Autodesk Inventor part; units mm, degrees
ref_plane "YZ Plane" through (0, 0, 0) normal (1, 0, 0) x (0, 1, 0)
ref_plane "XZ Plane" through (0, 0, 0) normal (0, 1, 0) x (-1, 0, 0)
ref_plane "XY Plane" through (0, 0, 0) normal (0, 0, 1) x (1, 0, 0)
sketch "Sketch2" plane through (0, 0, 0) normal (0, 1, 0) x (-1, 0, 0)
  circle A0 centre (0, 0) radius 30.16 construction
  line L0 (0, 0) -> (38.16, 0) construction
  line L1 (38.16, 38.16) -> (38.16, -38.16)
  line L2 (38.16, 38.16) -> (-30.16, 38.16)
  line L3 (38.16, -38.16) -> (-30.16, -38.16)
  circle A1 centre (27.211, 31.78) radius 2.55
  circle A2 centre (27.211, -31.78) radius 2.55
  circle A3 centre (0, 0) radius 2.55
  line L4 (-30.16, 38.16) -> (-30.16, -38.16)
  dimension "d12" = 60.32
  dimension "d13" = 38.16
  dimension "d14" = 76.32
  dimension "d15" = 5.1
  dimension "d17" = 6.38
  dimension "d18" = 10.949
  dimension "d19" = 5.1
extrude "Extrusion2" add sketch "Sketch2" along normal blind 3
fillet "Fillet2" radius 3 2 edges at (-38.16, 1.5, 38.16) (-38.16, 1.5, -38.16)
properties part number "Tapa" material "PMMA Plastic"
Source: CAD feature listing. Evaluate the final solid. Frame: model axes, mm. Round coordinates to 2 decimals unless told otherwise and drop trailing zeros. Order: outer loops, then holes, each group sorted by start corner. A loop starts at its lowest first (then second) coordinate and runs counter-clockwise, first axis right, second up. Notation, with made-up numbers: (78.25, -31) - (118.25, -31) arc R26 cw to (118.25, -8) - close; hole circle Ø10 at (24.25, 46). An arc over 180 degrees is marked (long way). Use a Markdown table: item, result. Add a question column.
1. First-contact query: pin 1 (4.5 mm diameter, centred on x = -27.211, z = 31.78, fed in from +Y). Flat tip, straight axial feed; report the tip coordinate or a pass-through.
2. Mould query, pull axis Z, two halves, no side actions, for faces 1 (the cylindrical face through (-37.3, 1.52, 37.26)), 2 (the cylindrical face through (-37.26, 1.52, -37.3)), 3 (the flat face through (30.16, 1, 1)), 4 (the cylindrical face through (-25.33, 1.48, 30.06)). Classes: +Z half, -Z half, draft (parallel to the pull), parting line (faces both ways), or undercut.
3. Line query: probe 1 along Z at (x, y) = (0, 0.95); probe 2 along Z at (x, y) = (-25, 1.3); probe 3 along Z at (x, y) = (-1, 2.45). Output: solid intervals per line, ascending.
4. Section query A-A (z = 31.78). Return the cut outline in (x, y), then the cut area to 3 significant figures.
Derived:
| question | item | result |
|---|---|---|
| 1 | pin 1 | through |
| 2 | face 1 | +Z half |
| 2 | face 2 | -Z half |
| 2 | face 3 | draft |
| 2 | face 4 | undercut |
| 3 | probe 1 | -38.16 to -2.55, 2.55 to 38.16 |
| 3 | probe 2 | -38.16 to -33.05, -30.51 to 30.51, 33.05 to 38.16 |
| 3 | probe 3 | -38.16 to -2.35, 2.35 to 38.16 |
| 4 | outline | (-38.16, 0) - (-29.76, 0) - (-29.76, 3) - (-38.16, 3) - close; (-24.66, 0) - (30.16, 0) - (30.16, 3) - (-24.66, 3) - close |
| 4 | area | 190 mm2 |
